```python
from build123d import *

# Parameters (mm, degrees)
SKETCH1_W           = 323
SKETCH1_H           = 83
BOSS_EXTRUDE1_DEPTH = 3
SKETCH2_W           = 20
SKETCH2_H           = 12
CUT_EXTRUDE1_DEPTH  = 10
SKETCH4_R           = 1.75
CUT_EXTRUDE2_DEPTH  = 4


with BuildPart() as part:
    # Sketch1 → Boss-Extrude1 (new body)
    with BuildSketch(Plane.XY):
        Rectangle(SKETCH1_W, SKETCH1_H)
    extrude(amount=BOSS_EXTRUDE1_DEPTH)

    # Sketch2 → Cut-Extrude1 (cut)
    with BuildSketch(Plane(origin=(0, 0, 0), x_dir=(-1, 0, 0), z_dir=(0, 0, -1))):
        with Locations((-121.5, -35.5)):
            Rectangle(SKETCH2_W, SKETCH2_H)
    extrude(amount=-CUT_EXTRUDE1_DEPTH, mode=Mode.SUBTRACT)

    # Sketch4 → Cut-Extrude2 (cut, through all)
    with BuildSketch(Plane(origin=(0, 0, 0), x_dir=(-1, 0, 0), z_dir=(0, 0, -1))):
        with Locations((152.5, -21.5)):
            Circle(SKETCH4_R)
        with Locations((-152.5, -21.5)):
            Circle(SKETCH4_R)
        with Locations((152.5, 21.5)):
            Circle(SKETCH4_R)
        with Locations((-152.5, 21.5)):
            Circle(SKETCH4_R)
    extrude(amount=-CUT_EXTRUDE2_DEPTH, mode=Mode.SUBTRACT)


solid = part.part
```
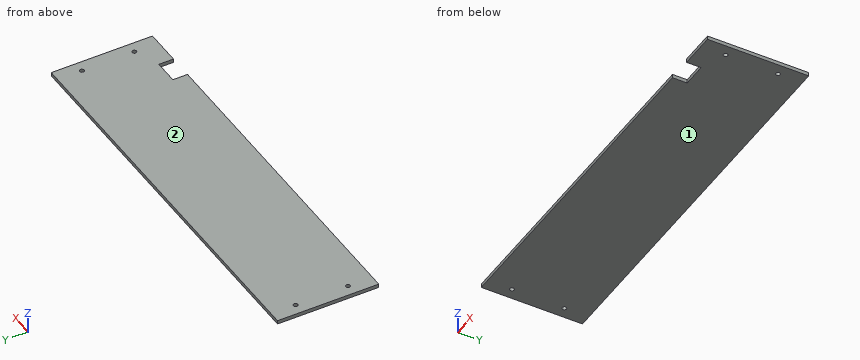
Build history of the part. All positions in model axes, mm. Face numbers are marked on the shaded views. Give positions to 0.01 mm unless a question says otherwise; leave off trailing zeros.
1) Probe line 1 along Y through (x, z) = (152.5, 1.35); line 2 along X through (y, z) = (-30, 2.4). List the from-to ranges inside material, lowest first.
Values follow:
line 1: y = -41.5 to -23.25, -19.75 to 19.75, 23.25 to 41.5
line 2: x = -161.5 to 111.5, 131.5 to 161.5
2) Two-plate mould, pull along Z, no slides. Class the marked faces 1 and 2: released by +Z, released by -Z, zero draft, split by the parting line, or undercut.
Values follow:
face 1: released by -Z
face 2: released by +Z
3) Drop a flat-ended pin along its axis: P1, Ø1.5, axis at x = 124, z = 1.5, coming from the -Y side. Give the stop position or say it passes through.
Values follow:
P1: stops at y = -29.5
